Geometry check sheet. Reference: the model listing, model coordinates, mm. Face numbers are marked on the shaded views. Give positions to 0.01 mm unless a question says otherwise; leave off trailing zeros. Loops run counter-clockwise (first coordinate to the right, second up) from the corner with the lowest first, then second, coordinate; pieces in that order, holes last. Notation, with made-up numbers: (6.5, -25.5) - (16.5, -25.5) arc R26 cw to (16.5, 2.5) - close; hole circle Ø10 at (82.25, 34). An arc over 180 degrees is marked (long way). Use a Markdown table: item, result. Add a question column.
1. Cross-section at C-C on y = 99.5. Enter the section's corners in (x, z).
2. Cross-section at B-B on x = -20. Enter the section's corners in (y, z).
3. Cross-section at D-D on y = 36. Enter the section's corners in (x, z), and give its area (3 significant figures).
4. Depth check by flat-ended pin: P1, Ø4, axis at x = -27.5, z = -51, coming from the -Y side; P2, Ø1, axis at x = -76, y = 41.5, coming from the -Z side; P3, Ø4, axis at x = 22.5, y = 47.5, coming from the +Z side; P4, Ø3, axis at y = 32.5, z = 36.5, coming from the -X side (3 decimals). Enter the tip coordinate at first touch or a pass-through.
5. Cross-section at A-A on z = 0. Enter the section's corners in (x, y).
6. Material ranges on L1, parallel to X at y = 96, z = 0; L2, parallel to Z at x = -20, y = 81.5; L3, parallel to Z at x = -20, y = 51, recorded low to high.
7. Draft check along Z on the marked faces 1, 2 and 3. Enter one of: pulls with the +Z half, pulls with the -Z half, needs draft (parallel to the pull), parting line crosses it, or undercut.
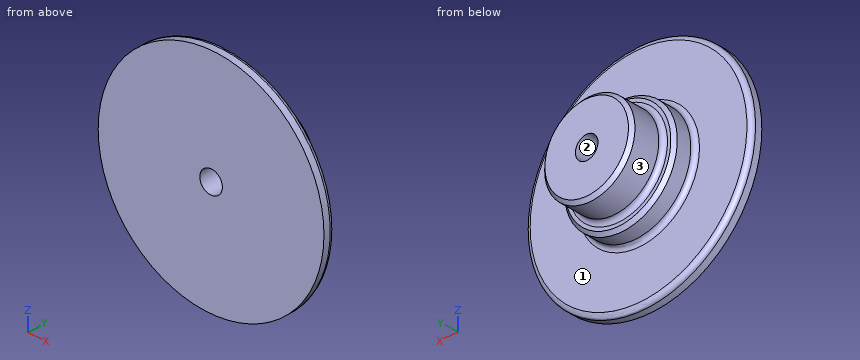
from build123d import *

# Parameters (mm, degrees)
FILLET4_R     = 8
CHAMFER5_SIZE = 6
FILLET5_R     = 8


with BuildPart() as part:
    # Sketch1 → Revolve5 (revolve)
    with BuildSketch(Plane.XY):
        Polygon((180, 0), (0, 0), (0, 120), (60, 120), (60, 60), (80, 60), (80, 20), (180, 20), align=None)
    revolve(axis=Axis((-20, 0, 0), (0, 1, 0)))

    # Fillet4
    fillet4_edges = [part.edges().sort_by_distance(p)[0] for p in [
        (-220, 20, 0),
    ]]
    fillet(fillet4_edges, radius=FILLET4_R)

    # Chamfer5
    chamfer5_edges = [part.edges().sort_by_distance(p)[0] for p in [
        (-120, 60, 0),
        (-100, 120, 0),
    ]]
    chamfer(chamfer5_edges, length=CHAMFER5_SIZE)

    # Fillet5
    fillet5_edges = [part.edges().sort_by_distance(p)[0] for p in [
        (-120, 20, 0),
        (-100, 60, 0),
    ]]
    fillet(fillet5_edges, radius=FILLET5_R)


solid = part.part
Values found:
| question | item | result |
|---|---|---|
| 1 | outline | circle Ø160 at (-20, 0); hole circle Ø40 at (-20, 0) |
| 2 | outline | (0, -200) - (12, -200) arc R8 ccw to (20, -192) - (20, -108) arc R8 cw to (28, -100) - (54, -100) - (60, -94) - (60, -88) arc R8 cw to (68, -80) - (114, -80) - (120, -74) - (120, -20) - (0, -20) - close; (0, 20) - (120, 20) - (120, 74) - (114, 80) - (68, 80) arc R8 cw to (60, 88) - (60, 94) - (54, 100) - (28, 100) arc R8 cw to (20, 108) - (20, 192) arc R8 ccw to (12, 200) - (0, 200) - close |
| 3 | outline | circle Ø200 at (-20, 0); hole circle Ø40 at (-20, 0) |
| 3 | area | 30,200 mm2 |
| 4 | P1 | stops at y = 0 |
| 4 | P2 | stops at z = -83.19 |
| 4 | P3 | stops at z = 91.43 |
| 4 | P4 | stops at x = -113.675 |
| 5 | outline | (-220, 0) - (-40, 0) - (-40, 120) - (-94, 120) - (-100, 114) - (-100, 68) arc R8 cw to (-108, 60) - (-114, 60) - (-120, 54) - (-120, 28) arc R8 cw to (-128, 20) - (-212, 20) arc R8 ccw to (-220, 12) - close; (0, 0) - (180, 0) - (180, 12) arc R8 ccw to (172, 20) - (88, 20) arc R8 cw to (80, 28) - (80, 54) - (74, 60) - (68, 60) arc R8 cw to (60, 68) - (60, 114) - (54, 120) - (0, 120) - close |
| 6 | L1 | x = -100 to -40, 0 to 60 |
| 6 | L2 | z = -80 to -20, 20 to 80 |
| 6 | L3 | z = -100 to -20, 20 to 100 |
| 7 | face 1 | needs draft |
| 7 | face 2 | undercut |
| 7 | face 3 | parting line crosses it |
